from build123d import *

# Parameters (mm, degrees)
EXTRUDE_1_DEPTH     = 57.7
EXTRUDE_2_DEPTH     = 30.8
SKETCH_5_R          = 4
CUT_EXTRUDE_1_DEPTH = 15
FILLET_1_R          = 10
SKETCH_6_W          = 6
SKETCH_6_H          = 1.5
EXTRUDE_3_DEPTH     = 6
EXTRUDE_START       = -37
SKETCH_6_3_W        = 6
SKETCH_6_3_H        = 1.5
EXTRUDE_4_DEPTH     = 6
SKETCH_7_R          = 2
CUT_EXTRUDE_2_DEPTH = 6
SKETCH_8_W          = 14.5
SKETCH_8_H          = 25.5
CUT_EXTRUDE_3_DEPTH = 2
CUT_EXTRUDE_START   = -26.9
CUT_EXTRUDE_4_DEPTH = 26.9
CUT_EXTRUDE_5_DEPTH = 44.487239508
SKETCH_11_W         = 6
SKETCH_11_H         = 6
CUT_EXTRUDE_6_DEPTH = 10


with BuildPart() as part:
    # 스케치1 → 보스-돌출1 (new body)
    with BuildSketch(Plane.XY):
        with BuildLine():
            Line((-13.5, 0), (-18.5, 0))
            Line((-18.5, 0), (-18.5, -18.5))
            Line((-18.5, -18.5), (18.5, -18.5))
            Line((18.5, -18.5), (18.5, 0))
            Line((18.5, 0), (13.5, 0))
            ThreePointArc((13.5, 0), (0, -13.5), (-13.5, 0))
        make_face()
    extrude(amount=-EXTRUDE_1_DEPTH)

    # 스케치3 → 보스-돌출2 (add)
    with BuildSketch(Plane.XY.offset(-26.9)):
        with BuildLine():
            Line((-13.5, 0), (-11.5, 0))
            ThreePointArc((-11.5, 0), (0, -11.5), (11.5, 0))
            Line((11.5, 0), (13.5, 0))
            ThreePointArc((13.5, 0), (0, -13.5), (-13.5, 0))
        make_face()
    extrude(amount=-EXTRUDE_2_DEPTH)

    # 스케치5 → 컷-돌출1 (cut)
    with BuildSketch(Plane.ZY.offset(18.5)):
        with Locations((-21.9, 0)):
            Circle(SKETCH_5_R)
    extrude(amount=-CUT_EXTRUDE_1_DEPTH, mode=Mode.SUBTRACT)

    # 필렛1
    fillet_1_edges = [part.edges().sort_by_distance(p)[0] for p in [
        (18.5, -18.5, -28.85),
        (-18.5, -18.5, -28.85),
    ]]
    fillet(fillet_1_edges, radius=FILLET_1_R)

    # 스케치6 → 보스-돌출3 (add)
    with BuildSketch(Plane(origin=(18.5, 0, 0), x_dir=(0, 0, -1), z_dir=(1, 0, 0))):
        with Locations((52.7, -0.75)):
            Rectangle(SKETCH_6_W, SKETCH_6_H)
        with Locations((5, -0.75)):
            Rectangle(SKETCH_6_W, SKETCH_6_H)
    extrude(amount=EXTRUDE_3_DEPTH)

    # 스케치6<3> → 보스-돌출4 (add)
    with BuildSketch(Plane(origin=(18.5, 0, 0), x_dir=(0, 0, -1), z_dir=(1, 0, 0)).offset(EXTRUDE_START)):
        with Locations((52.7, -0.75)):
            Rectangle(SKETCH_6_3_W, SKETCH_6_3_H)
        with Locations((5, -0.75)):
            Rectangle(SKETCH_6_3_W, SKETCH_6_3_H)
    extrude(amount=-EXTRUDE_4_DEPTH)

    # 스케치7 → 컷-돌출2 (cut)
    with BuildSketch(Plane(origin=(0, 0, 0), x_dir=(1, 0, 0), z_dir=(0, 1, 0))):
        with Locations(Location((21.5, 5, 0), (0, 0, 270))):
            Circle(SKETCH_7_R)
        with Locations(Location((21.5, 52.7, 0), (0, 0, 270))):
            Circle(SKETCH_7_R)
        with Locations(Location((-21.5, 5, 0), (0, 0, 180))):
            Circle(SKETCH_7_R)
        with Locations((-21.5, 52.7)):
            Circle(SKETCH_7_R)
    extrude(amount=-CUT_EXTRUDE_2_DEPTH, mode=Mode.SUBTRACT)

    # 스케치8 → 컷-돌출3 (cut)
    with BuildSketch(Plane.XZ.offset(18.5)):
        with Locations((0, -42.95)):
            Rectangle(SKETCH_8_W, SKETCH_8_H)
    extrude(amount=-CUT_EXTRUDE_3_DEPTH, mode=Mode.SUBTRACT)

    # 스케치9 → 컷-돌출4 (cut)
    with BuildSketch(Plane.XY.offset(CUT_EXTRUDE_START)):
        with BuildLine():
            Line((-13.5, 0), (-13.75, 0))
            ThreePointArc((-13.75, 0), (0, -13.75), (13.75, 0))
            Line((13.75, 0), (13.5, 0))
            ThreePointArc((13.5, 0), (0, -13.5), (-13.5, 0))
        make_face()
    extrude(amount=CUT_EXTRUDE_4_DEPTH, mode=Mode.SUBTRACT)

    # 스케치10 → 컷-돌출5 (cut, through all)
    with BuildSketch(Plane.XY.offset(-26.9)):
        with BuildLine():
            ThreePointArc((11.5, 0), (0, -11.5), (-11.5, 0))
            Line((-11.5, 0), (-12.5, 0))
            ThreePointArc((-12.5, 0), (0, -12.5), (12.5, 0))
            Line((12.5, 0), (11.5, 0))
        make_face()
    extrude(amount=-CUT_EXTRUDE_5_DEPTH, mode=Mode.SUBTRACT)

    # 스케치11 → 컷-돌출6 (cut)
    with BuildSketch(Plane.XZ.offset(1.5)):
        with Locations((21.5, -5)):
            Rectangle(SKETCH_11_W, SKETCH_11_H)
    extrude(amount=-CUT_EXTRUDE_6_DEPTH, mode=Mode.SUBTRACT)


solid = part.part
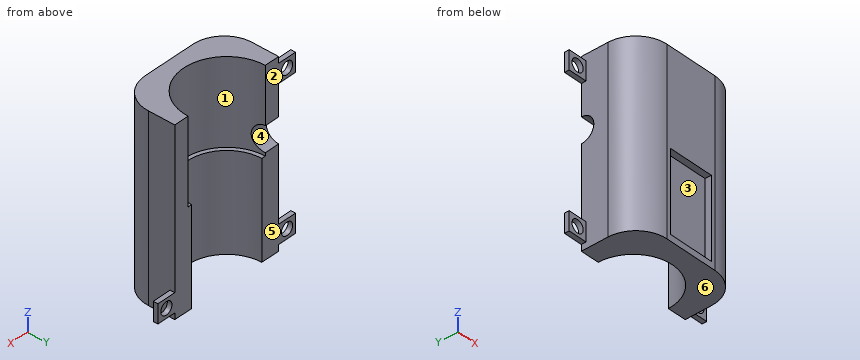
Read the model definition and answer for the solid it produces. Units are mm, in the model's axes. Face numbers are marked on the shaded views. A direction names the side the tool comes from. Coordinates: 2 decimals unless noted, no trailing zeros. Loops run counter-clockwise (first coordinate to the right, second up) from the corner with the lowest first, then second, coordinate; pieces in that order, holes last.
Q1. The part is cut by section D-D on y = -6.75. Write down the section's boundary in (x, z).
Q2. The mould has two halves that part along Z. Classify the marked faces 4, 5 and 6: +Z half, -Z half, draft (parallel to the pull), parting line (faces both ways), or undercut.
Q3. Each of these flat-tipped pins is pushed along its axis until it touches: pin 1 Ø1.6 at (x, y) = (22, -1) entering from +Z; pin 2 Ø4.5 at (x, z) = (-1, -40.5) entering from -Y; pin 3 Ø5 at (x, z) = (-21.5, -52.7) entering from -Y; pin 4 Ø1 at (x, y) = (-8.5, -6) entering from +Z. Where does it stop, or does it pass through?
Q4. Consider probe 1 along X at (y, z) = (-0.4, -52.7); probe 2 along Z at (x, y) = (-21.5, -1.15); probe 3 along Z at (x, y) = (-9, -10). Determine where each line is inside the solid, lowest interval first.
Q5. The part is cut by section A-A on x = 21.5. Write down the section's boundary in (y, z).
Q6. The part is cut by section C-C on x = -21.5. Write down the section's boundary in (y, z).
Q7. Which of the six approach directions +Z, -Z, +X, -X, +Y, -Y give full straight-line access (tool end or side, diameter ignored) to the marked faces 1, 2 and 3?
Q8. The part is cut by section B-B on z = -5. Write down the section's boundary in (x, y), and give its area (3 significant figures).
Results below:
1. outline: (-18.5, -57.7) - (-10.52, -57.7) - (-10.52, -26.9) - (-11.98, -26.9) - (-11.98, 0) - (-18.5, 0) - close; (10.52, -57.7) - (18.5, -57.7) - (18.5, 0) - (11.98, 0) - (11.98, -26.9) - (10.52, -26.9) - close
2. face 4: undercut
2. face 5: draft
2. face 6: -Z half
3. pin 1: stops at z = -49.7
3. pin 2: stops at y = -16.5
3. pin 3: stops at y = -1.5
3. pin 4: passes through
4. probe 1: x = -24.5 to -23.5, -19.5 to -12.49, 12.49 to 19.5, 23.5 to 24.5
4. probe 2: z = -55.7 to -54.7, -50.7 to -49.7, -8 to -7, -3 to -2
4. probe 3: z = -57.7 to -26.9
5. outline: (-1.5, -55.7) - (0, -55.7) - (0, -54.7) - (-1.5, -54.7) - close; (-1.5, -50.7) - (0, -50.7) - (0, -49.7) - (-1.5, -49.7) - close
6. outline: (-1.5, -55.7) - (0, -55.7) - (0, -54.7) - (-1.5, -54.7) - close; (-1.5, -50.7) - (0, -50.7) - (0, -49.7) - (-1.5, -49.7) - close; (-1.5, -8) - (0, -8) - (0, -7) - (-1.5, -7) - close; (-1.5, -3) - (0, -3) - (0, -2) - (-1.5, -2) - close
7. face 1: +Z, +Y
7. face 2: +Z, -Z, +X, -X, +Y
7. face 3: -Y
8. outline: (-24.5, -1.5) - (-23.5, -1.5) - (-23.5, 0) - (-24.5, 0) - close; (-19.5, -1.5) - (-18.5, -1.5) - (-18.5, -8.5) arc R10 ccw to (-8.5, -18.5) - (8.5, -18.5) arc R10 ccw to (18.5, -8.5) - (18.5, 0) - (13.75, 0) arc R13.75 cw to (-13.75, 0) - (-19.5, 0) - close
8. area: 348 mm2
